Job drawing, mm, ordinate dimensions from the low corner. One solid piece. A direction names the side the tool comes from. Coordinates: 2 decimals unless noted, no trailing zeros. Loops run counter-clockwise (first coordinate to the right, second up) from the corner with the lowest first, then second, coordinate; pieces in that order, holes last. Notation, with made-up numbers: (56, 10.5) - (66, 10.5) arc R32 ccw to (66, 44.5) - close; hole circle Ø4 at (-7, -35.5). An arc over 180 degrees is marked (long way). Use a Markdown table: item, result. Add a question column.
1. 3-axis set-ups, long thin cutter, end or side, ignore diameter. For the marked faces 1, 2, 3 and 4: which of +Z, -Z, +X, -X, +Y, -Y reach the whole face in a straight line?
2. Wall check: probe 1 along X at (y, z) = (26.5, 6.25); probe 2 along Z at (x, y) = (19, 25); probe 3 along X at (y, z) = (5, 30). Give the ranges that are in metal, low to high. Write a range as [from, to].
3. Drop flat-ended pins along their axis: pin 1 (7 mm diameter, centred on x = 20.5, y = 14, fed in from -Z); pin 2 (3 mm diameter, centred on x = 19.25, z = 53.75, fed in from +Y); pin 3 (5.5 mm diameter, centred on x = 12.5, z = 30, fed in from +Y). Give the stop position or say it passes through.
4. Pull direction X, two halves, no side cores. Call the marked faces 5, 6 and 7: pulls with the +X half, pulls with the -X half, needs draft (parallel to the pull), parting line crosses it, or undercut.
5. Band-saw the part on D-D, the plane x = 12.5. Give the cut face in (y, z), plus the area to 3 significant figures.
6. Band-saw the part on C-C, the plane y = 17. Give the cut face in (x, z).
7. Band-saw the part on A-A, the plane y = 23.5. Give the cut face in (x, z), plus the area to 3 significant figures.
8. Band-saw the part on B-B, the plane z = 30. Give the cut face in (x, y), plus the area to 3 significant figures.
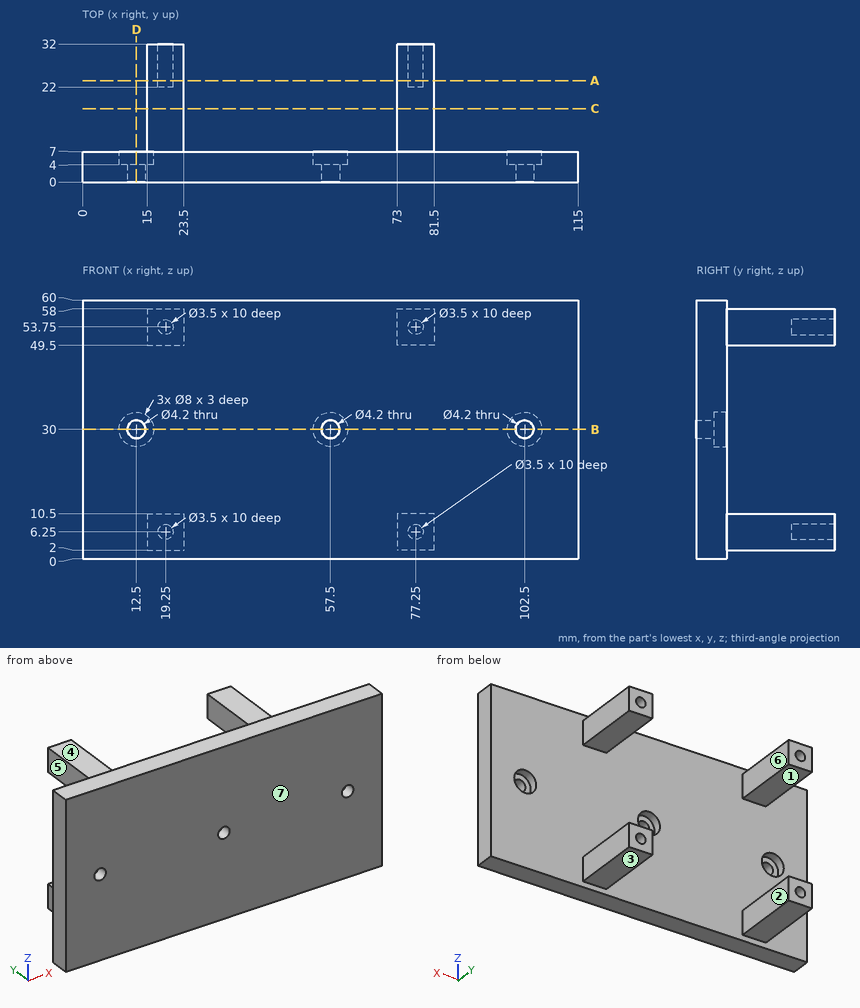
Geometry check:
| question | item | result |
|---|---|---|
| 1 | face 1 | +X, -X, +Y |
| 1 | face 2 | +Z, -Z, +Y |
| 1 | face 3 | -Z, +X, -X, +Y |
| 1 | face 4 | +Z, +X, -X, +Y |
| 2 | probe 1 | x = [15, 17.5], [21, 23.5], [73, 75.5], [79, 81.5] |
| 2 | probe 2 | z = [2, 4.52], [7.98, 10.5], [49.5, 52.02], [55.48, 58] |
| 2 | probe 3 | x = [0, 8.5], [16.5, 53.5], [61.5, 98.5], [106.5, 115] |
| 3 | pin 1 | stops at z = 2 |
| 3 | pin 2 | stops at y = 22 |
| 3 | pin 3 | stops at y = 4 |
| 4 | face 5 | pulls with the -X half |
| 4 | face 6 | undercut |
| 4 | face 7 | needs draft |
| 5 | outline | (0, 0) - (7, 0) - (7, 26) - (4, 26) - (4, 27.9) - (0, 27.9) - close; (0, 32.1) - (4, 32.1) - (4, 34) - (7, 34) - (7, 60) - (0, 60) - close |
| 5 | area | 379 mm^2 |
| 6 | outline | (15, 2) - (23.5, 2) - (23.5, 10.5) - (15, 10.5) - close; (15, 49.5) - (23.5, 49.5) - (23.5, 58) - (15, 58) - close; (73, 2) - (81.5, 2) - (81.5, 10.5) - (73, 10.5) - close; (73, 49.5) - (81.5, 49.5) - (81.5, 58) - (73, 58) - close |
| 7 | outline | (15, 2) - (23.5, 2) - (23.5, 10.5) - (15, 10.5) - close; (15, 49.5) - (23.5, 49.5) - (23.5, 58) - (15, 58) - close; (73, 2) - (81.5, 2) - (81.5, 10.5) - (73, 10.5) - close; (73, 49.5) - (81.5, 49.5) - (81.5, 58) - (73, 58) - close; hole circle Ø3.5 at (19.25, 6.25); hole circle Ø3.5 at (19.25, 53.75); hole circle Ø3.5 at (77.25, 6.25); hole circle Ø3.5 at (77.25, 53.75) |
| 7 | area | 251 mm^2 |
| 8 | outline | (0, 0) - (10.4, 0) - (10.4, 4) - (8.5, 4) - (8.5, 7) - (0, 7) - close; (14.6, 0) - (55.4, 0) - (55.4, 4) - (53.5, 4) - (53.5, 7) - (16.5, 7) - (16.5, 4) - (14.6, 4) - close; (59.6, 0) - (100.4, 0) - (100.4, 4) - (98.5, 4) - (98.5, 7) - (61.5, 7) - (61.5, 4) - (59.6, 4) - close; (104.6, 0) - (115, 0) - (115, 7) - (106.5, 7) - (106.5, 4) - (104.6, 4) - close |
| 8 | area | 683 mm^2 |
